```python
from build123d import *

# Parameters (mm, degrees)
F0_W     = 52.1929860115
F0_H     = 5.8492124081
F1_DEPTH = 51.4541193843
F2_W     = 52.1929860115
F2_H     = 6.8990886211
F3_DEPTH = 33.7024219334
F4_W     = 52.2046461701
F4_H     = 5.920117721
F5_DEPTH = 44.953584671
F6_R     = 5.08
F7_R     = 5.08


with BuildPart() as f1:
    # F0 (on Top) → F1 (new body)
    with BuildSketch(Plane.XY):
        with Locations((-0.8998662233, 36.52010113)):
            Rectangle(F0_W, F0_H)
    extrude(amount=F1_DEPTH)

    # F2 (on Front) → F3 (join)
    with BuildSketch(Plane.XZ):
        with Locations((-1.0498464108, 3.4495443106)):
            Rectangle(F2_W, F2_H)
    extrude(amount=-F3_DEPTH)

    # F4 (on Top) → F5 (join)
    with BuildSketch(Plane.XY):
        with Locations((-1.1427812278, 2.9600588605)):
            Rectangle(F4_W, F4_H)
    extrude(amount=-F5_DEPTH)

    # F6
    f6_edges = [f1.edges().sort_by_distance(p)[0] for p in [
        (-1.142781, 5.920118, -44.953585),
    ]]
    fillet(f6_edges, radius=F6_R)

    # F7
    f7_edges = [f1.edges().sort_by_distance(p)[0] for p in [
        (-0.899866, 33.595495, 51.454119),
    ]]
    fillet(f7_edges, radius=F7_R)


solid = f1.part
```
Here's how the part is built. I have some questions about the finished solid (model axes, mm). A direction names the side the tool comes from. Give positions to 0.01 mm unless a question says otherwise; leave off trailing zeros. Loops run counter-clockwise (first coordinate to the right, second up) from the corner with the lowest first, then second, coordinate; pieces in that order, holes last. Notation, with made-up numbers: (53.25, 87.5) -> (71.25, 87.5) arc R23 cw to (71.25, 114.5) -> close; hole circle Ø2 at (3, 2.25). An arc over 180 degrees is marked (long way). Use one line per item in the form item = value. Start each with the question number.
1) Imagine slicing it at B-B (z = 30). Please give me the cut outline in (x, y), then the cut area to 3 significant figures.
2) Imagine slicing it at C-C (y = 13). Please give me the cut outline in (x, z), then the cut area to 3 significant figures.
3) Imagine slicing it at A-A (x = -17). Please give me the cut outline in (y, z), then the cut area to 3 significant figures.
4) Please list where these lines run through material, in increasing order: line 1 along Z through (x, y) = (1, 15); line 2 along Y through (x, z) = (8, -27.5); line 3 along Y through (x, z) = (15, 37.5).
5) For P1, Ø19.5, axis at x = 11.5, y = 28.5, coming from the -Z side; P2, Ø3, axis at y = 3, z = -24, coming from the +X side; P3, Ø6, axis at x = -20, z = 21.5, coming from the -Y side; P4, Ø1.5, axis at y = 29, z = 9, coming from the +X side, each with a flat end and sliding along its axis, tell me the tip position at first contact or that it passes through.
6) Which directions (+Z, -Z, +X, -X, +Y, -Y) give clear straight access to the entire face, cutting with the end or side of a thin tool? Please do faces 1 (the face through (25.047, 17, 3)), 2 (the face through (-2, 5.92, -20)), 3 (the face through (-27.146, 17, 3)), 4 (the face through (-27.245, 3, -22)), 5 (the face through (24.96, 3, -22)).
Check values:
q1.outline = (-27, 33.6) -> (25.2, 33.6) -> (25.2, 39.44) -> (-27, 39.44) -> close
q1.area = 305 mm^2
q2.outline = (-27.15, 0) -> (25.05, 0) -> (25.05, 6.9) -> (-27.15, 6.9) -> close
q2.area = 360 mm^2
q3.outline = (0, -44.95) -> (0.84, -44.95) arc R5.08 ccw to (5.92, -39.87) -> (5.92, 0) -> (39.44, 0) -> (39.44, 51.45) -> (38.68, 51.45) arc R5.08 ccw to (33.6, 46.37) -> (33.6, 6.9) -> (0, 6.9) -> close
q3.area = 788 mm^2
q4.line_1 = 0 to 6.9
q4.line_2 = 0 to 5.92
q4.line_3 = 33.6 to 39.44
q5.P1 = 0
q5.P2 = 24.96
q5.P3 = 33.6
q5.P4 = through
q6.face_1 = +Z, -Z, +X, -Y
q6.face_2 = -Z, +X, -X, +Y
q6.face_3 = +Z, -X, +Y, -Y
q6.face_4 = +Z, -Z, -X, +Y, -Y
q6.face_5 = -Z, +X, +Y, -Y
